Geometry check sheet. Reference: the model listing, model coordinates, mm. A direction names the side the tool comes from. Round coordinates to 2 decimals unless told otherwise and drop trailing zeros. Write each loop counter-clockwise with the first axis right and the second up, starting at its lowest first coordinate (ties: lowest second). Pieces come first, ordered by that corner, then holes. Notation, with made-up numbers: (-11.75, -35.75) -> (5.25, -35.75) arc R14 ccw to (5.25, -31.75) -> close; hole circle Ø5 at (13, 79). An arc over 180 degrees is marked (long way). Use a Markdown table: item, result.
```python
from build123d import *

# Parameters (mm, degrees)
FILLET1_R = 0.635
FILLET2_R = 0.254


with BuildPart() as part:
    # Sketch1 → Revolve1 (revolve)
    with BuildSketch(Plane.XY, mode=Mode.PRIVATE) as revolve1_sk:
        with BuildLine():
            Line((-0.8509, 8.0518), (-0.8509, 2.2098))
            Line((-0.8509, 2.2098), (0, 2.2098))
            Line((0, 2.2098), (0, 0))
            ThreePointArc((0, 0), (-3.193462918, 0.171947054), (-6.35, 0.6858))
            Line((-6.35, 0.6858), (-6.35, 2.2098))
            Line((-6.35, 2.2098), (-1.397, 2.2098))
            Line((-1.397, 2.2098), (-1.397, 8.0518))
            Line((-1.397, 8.0518), (-0.8509, 8.0518))
        make_face()
    revolve(revolve1_sk.sketch.rotate(Axis((0, 0, 0), (0, 1, 0)), 270), axis=Axis((0, 0, 0), (0, 1, 0)))

    # Fillet1
    fillet1_edges = [part.edges().sort_by_distance(p)[0] for p in [
        (0, 2.2098, 1.397),
        (0, 2.2098, 6.35),
        (0, 0.6858, 6.35),
    ]]
    fillet(fillet1_edges, radius=FILLET1_R)

    # Fillet2
    fillet2_edges = [part.edges().sort_by_distance(p)[0] for p in [
        (0, 8.0518, 1.397),
        (0, 8.0518, 0.8509),
    ]]
    fillet(fillet2_edges, radius=FILLET2_R)


solid = part.part
```
(1) Access from +Z, -Z, +X, -X, +Y, -Y to the whole of each face (thin tool, end or side, straight path). Record for faces 4 (the face through (-1.907, 1.391, -6.057)), 5 (the face through (0, 2.21, 0)).
A:
| item | result |
|---|---|
| face 4 | +Y, -Y |
| face 5 | +Y |
(2) Gauge pin test, flat ends, axial feed: pin 1 Ø1.4 at (x, z) = (0, 0) entering from +Y; pin 2 Ø3 at (x, z) = (-1.5, -2.5) entering from -Y; pin 3 Ø1 at (y, z) = (6, 0.5) entering from -X. Record the tip position at first contact, or that the pin passes through.
A:
| item | result |
|---|---|
| pin 1 | stops at y = 2.21 |
| pin 2 | stops at y = 0.03 |
| pin 3 | stops at x = -1.4 |
(3) Section check A-A on y = 4.75. Record the cut outline in (x, z), plus the area to 3 significant figures.
A:
| item | result |
|---|---|
| outline | circle Ø2.79 at (0, 0); hole circle Ø1.7 at (0, 0) |
| area | 3.86 mm2 |
(4) Thickness scan on line 1 (X direction, y = 3.95, z = 0); line 2 (Z direction, x = -0.5, y = 5.5); line 3 (Y direction, x = 0.5, z = 1.5). Record the ranges inside material, lowest first.
A:
| item | result |
|---|---|
| line 1 | x = -1.4 to -0.85, 0.85 to 1.4 |
| line 2 | z = -1.3 to -0.69, 0.69 to 1.3 |
| line 3 | y = 0.04 to 2.4 |
(5) Release check for a two-part mould opening along Z. For faces 1 (the face through (1.364, 5.356, 0.303)), 2 (the face through (-0.844, 4.965, 0.111)), 3 (the face through (-0.1, 2.21, -2.5)) record: +Z half, -Z half, draft (parallel to the pull), parting line (faces both ways), or undercut.
A:
| item | result |
|---|---|
| face 1 | parting line |
| face 2 | undercut |
| face 3 | draft |
